```python
from build123d import *

# Parameters (mm, degrees)
F0_W     = 101.6
F0_H     = 152.4
F1_DEPTH = 25.4
F3_DEPTH = 6.35
F2_W     = 51.8073203593
F2_H     = 24.3617037889
F4_DEPTH = 6.35
F5_R     = 5.08


with BuildPart() as f1:
    # F0 (on Top) → F1 (new body)
    with BuildSketch(Plane.XY):
        with Locations((1.0073203593, 31.0641650792)):
            Rectangle(F0_W, F0_H)
    extrude(amount=F1_DEPTH)

    # F2 (on face) → F3 (join)
    with BuildSketch(Plane.XY.offset(25.4)):
        Polygon((-49.7926796407, 107.2641650792), (-49.7926796407, 82.9024612904), (-8.9114280418, 82.9024612904), (0, 82.9024612904), (0, 107.2641650792), align=None)
    extrude(amount=F3_DEPTH)

    # F2 (on face) → F4 (join)
    with BuildSketch(Plane.XY.offset(25.4)):
        with Locations((25.9036601797, 95.0833131848)):
            Rectangle(F2_W, F2_H)
    extrude(amount=F4_DEPTH)

    # F5
    f5_edges = [f1.edges().sort_by_distance(p)[0] for p in [
        (-49.79268, 95.083313, 31.75),
        (1.00732, 82.902461, 31.75),
        (51.80732, 95.083313, 31.75),
        (1.00732, 107.264165, 31.75),
    ]]
    fillet(f5_edges, radius=F5_R)


solid = f1.part
```
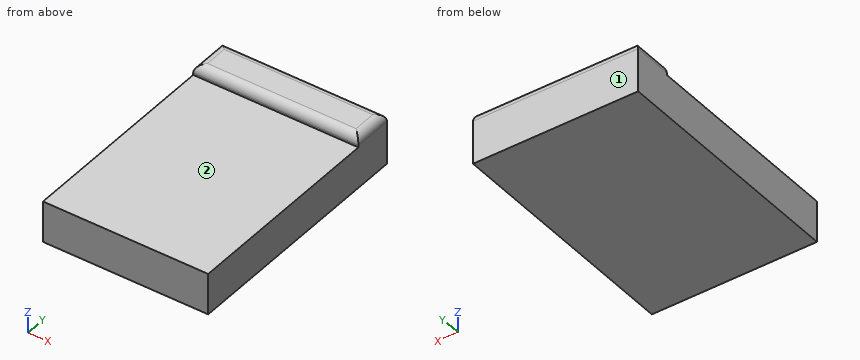
Source: CAD feature listing. Evaluate the final solid. Frame: model axes, mm. Face numbers are marked on the shaded views. A direction names the side the tool comes from. Round coordinates to 2 decimals unless told otherwise and drop trailing zeros. Loops run counter-clockwise (first coordinate to the right, second up) from the corner with the lowest first, then second, coordinate; pieces in that order, holes last.
1. Ray query, L1, parallel to Z at x = -33.5, y = 58.5; L2, parallel to Y at x = 15, z = 29. Return the intervals inside material, ascending.
2. Access query for the marked faces 1 and 2. Directions: +Z, -Z, +X, -X, +Y, -Y. A direction counts if a zero-diameter tool reaches every point of the face in a straight line with its end or side. Return the directions, or none.
3. Section query B-B on y = 5. Output: boundary loops of the cut face in (x, z), and give its area (3 significant figures).
4. Section query A-A on x = 39. Output: boundary loops of the cut face in (y, z).
5. Contact query for a flat-ended pin moving along its axis: pin 1 (5 mm diameter, centred on x = 32.5, y = 48, fed in from +Z). Output: stop coordinate, or through.
Answers below:
1. L1: z = 0 to 25.4
1. L2: y = 83.47 to 106.7
2. face 1: +Z, -Z, +X, -X, +Y
2. face 2: +Z, +X, -X, -Y
3. outline: (-49.79, 0) - (51.81, 0) - (51.81, 25.4) - (-49.79, 25.4) - close
3. area: 2,580 mm2
4. outline: (-45.14, 0) - (107.26, 0) - (107.26, 26.67) arc R5.08 ccw to (102.18, 31.75) - (87.98, 31.75) arc R5.08 ccw to (82.9, 26.67) - (82.9, 25.4) - (-45.14, 25.4) - close
5. pin 1: stops at z = 25.4
